from build123d import *

# Parameters (mm, degrees)
CYLINDER906_R     = 74
CYLINDER906_DEPTH = 32
BOX432_W          = 50
BOX432_H          = 6
BOX432_DEPTH      = 26
CHAMFER003_SIZE   = 20


with BuildPart() as obj1:
    # Cylinder906 → Cylinder906 (new body)
    with BuildSketch(Plane.XY.offset(50)):
        Circle(CYLINDER906_R)
    extrude(amount=CYLINDER906_DEPTH)


with BuildPart() as chamfer003:
    # Box432 → Box432 (new body)
    with BuildSketch(Plane(origin=(-112, -24, 56), x_dir=(1, 0, 0), z_dir=(0, 0, 1))):
        with Locations((25, 3)):
            Rectangle(BOX432_W, BOX432_H)
    extrude(amount=BOX432_DEPTH)

    # Cut406: cut obj1
    add(obj1.part, mode=Mode.SUBTRACT)

    # Chamfer003
    chamfer003_edges = [chamfer003.edges().sort_by_distance(p)[0] for p in [
        (-112, -21, 56),
    ]]
    chamfer(chamfer003_edges, length=CHAMFER003_SIZE)


solid = chamfer003.part
Read the model definition and answer for the solid it produces. Units are mm, in the model's axes. Round coordinates to 2 decimals unless told otherwise and drop trailing zeros. Order: outer loops, then holes, each group sorted by start corner. A loop starts at its lowest first (then second) coordinate and runs counter-clockwise, first axis right, second up.
1) The part is cut by section A-A on z = 73. Write down the section's boundary in (x, y).
2) Straight lines are drawn through the part: L1, parallel to X at y = -22.75, z = 69; L2, parallel to Z at x = -108, y = -21.75; L3, parallel to X at y = -21.75, z = 70.5. For each, find the intervals that lie inside material, in ascending order.
3) Flat-ended cylindrical pins translate along their axes: pin 1 (2 mm diameter, centred on y = -21, z = 71, fed in from -X); pin 2 (2 mm diameter, centred on x = -97, y = -19, fed in from -Z). Find the tip coordinate at first contact, or state that the pin passes through.
4) The part is cut by section C-C on y = -21.5. Write down the section's boundary in (x, z).
5) The part is cut by section D-D on y = -23.5. Write down the section's boundary in (x, z), plus the area to 3 significant figures.
6) The part is cut by section B-B on x = -109. Write down the section's boundary in (y, z).
Resolved:
1. outline: (-109, -24) - (-70, -24) arc R74 cw to (-71.78, -18) - (-109, -18) - close
2. L1: x = -105 to -70.42
2. L2: z = 72 to 82
2. L3: x = -106.5 to -70.73
3. pin 1: stops at x = -108
3. pin 2: stops at z = 60
4. outline: (-112, 76) - (-92, 56) - (-70.81, 56) - (-70.81, 82) - (-112, 82) - close
5. outline: (-112, 76) - (-92, 56) - (-70.17, 56) - (-70.17, 82) - (-112, 82) - close
5. area: 888 mm2
6. outline: (-24, 73) - (-18, 73) - (-18, 82) - (-24, 82) - close
